CAD build for the part. Positions are in the model's coordinates, mm. Give positions to 0.01 mm unless a question says otherwise; leave off trailing zeros. Write each loop counter-clockwise with the first axis right and the second up, starting at its lowest first coordinate (ties: lowest second). Pieces come first, ordered by that corner, then holes. Notation, with made-up numbers: (82.25, 3.25) - (89.25, 3.25) arc R13 cw to (89.25, 8.25) - close; hole circle Ø3 at (17, -25). An arc over 180 degrees is marked (long way). Answer as a JSON object with one key per item and string values.
Solid Edge part; units mm, degrees
sketch "Sketch1" plane through (0, 0, 0) normal (0, -1, 0) x (1, 0, 0)
  arc A0 (80, 427.0462) -> (149.1404, 208.2529) centre (454.9956, 425.2266) ccw
  line L0 (149.1404, 28.2529) -> (149.1404, 208.2529)
  line L1 (-150.8596, 28.2529) -> (149.1404, 28.2529)
  line L2 (-150.8596, 28.2529) -> (-150.8596, 208.8033)
  arc A1 (-80, 427.0462) -> (-150.8596, 208.8033) centre (-454.9983, 428.1766) cw
  arc A2 (-80, 427.0462) -> (80, 427.0462) centre (0, 427.0462) cw
extrude "ProtrusioneEstrusa_1" add sketch "Sketch1" along normal mid plane 10
fillet "Rotondo_1" radius 100 2 edges at (149.1404, 0, 208.2529) (-150.8596, 0, 208.8033)
sketch "Sketch2" plane through (-0.8596, -5, 267.6495) normal (0, -1, 0) x (1, 0, 0)
  circle A0 centre (0.8596, 159.3967) radius 10.5
extrude "Cutout1" cut sketch "Sketch2" against normal through all
properties material "Policarbonato"
Item 1: Cut at C-C (z = 301). Give the cut face in (x, y), and give its area (3 significant figures).
Entries:
{"outline": "(-102.22, -5) - (101.17, -5) - (101.17, 5) - (-102.22, 5) - close", "area": "2,030 mm2"}
Item 2: Cut at D-D (x = 85.5). Give the cut face in (y, z).
Entries:
{"outline": "(-5, 28.25) - (5, 28.25) - (5, 361.21) - (-5, 361.21) - close"}
Item 3: Probe line 1 (Z direction, x = 0, y = 2.5); line 2 (X direction, y = -1, z = 345); line 3 (X direction, y = -0.5, z = 396). List the from-to ranges inside material, lowest first. Write a range as from..to.
Entries:
{"line 1": "28.25..416.55, 437.55..507.05", "line 2": "-89.34..88.68", "line 3": "-81.38..81.14"}
Item 4: Flat gauge pins, fed straight in: P1, Ø5, axis at y = -1, z = 365, coming from the -X side; P2, Ø5, axis at y = -3, z = 407, coming from the +X side. Where does each tip first touch, or does it go through?
Entries:
{"P1": "x = -85.79", "P2": "x = 80.57"}
Item 5: Cut at B-B (x = 0). Give the cut face in (y, z).
Entries:
{"outline": "(-5, 28.25) - (5, 28.25) - (5, 416.55) - (-5, 416.55) - close; (-5, 437.55) - (5, 437.55) - (5, 507.05) - (-5, 507.05) - close"}
Item 6: Mould opens along X. For faces 1 (the flat face through (1, 5, 211)), 2 (the flat face through (-150.86, 0, 102)), 3 (the cylindrical face through (-1.367, -0.07, 437.457)) say: +X half, -X half, draft (parallel to the pull), parting line (faces both ways), or undercut.
Entries:
{"face 1": "draft", "face 2": "-X half", "face 3": "undercut"}
Item 7: Cut at A-A (y = 3.5). Give the cut face in (x, z), and give its area (3 significant figures).
Entries:
{"outline": "(-150.86, 28.25) - (149.14, 28.25) - (149.14, 178.43) arc R100 ccw to (134.58, 230.39) arc R375 cw to (80, 427.05) arc R80 ccw to (-80, 427.05) arc R375 cw to (-135.94, 231.13) arc R100 ccw to (-150.86, 178.58) - close; hole circle Ø21 at (0, 427.05)", "area": "108,000 mm2"}
